Source: CAD feature listing. Evaluate the final solid. Frame: model axes, mm. A direction names the side the tool comes from. Coordinates: 2 decimals unless noted, no trailing zeros. Order: outer loops, then holes, each group sorted by start corner. A loop starts at its lowest first (then second) coordinate and runs counter-clockwise, first axis right, second up.
```python
from build123d import *
from build123d import SkipClean  # not in build123d's __all__

# Parameters (mm, degrees)
F1_DEPTH    = 28
F2_T1_DEPTH = 28
F2_T3_DEPTH = 31.2745707181
F3_R        = 14
F4_DEPTH    = 4
F6_DEPTH    = 2.5
F7_R        = 3.25
F8_DEPTH    = 31.3042238242
F9_R        = 7.5
F10_DEPTH   = 24.8042238242
F11_R       = 6.5
F12_DEPTH   = 4
F13_W       = 4
F13_H       = 21.4542382136
F14_DEPTH   = 2.5
F15_W       = 14
F15_H       = 21.4542382136
F16_DEPTH   = 1.2
F18_DEPTH   = 14


# Not quite as in the source:
# - a fillet or chamfer that OpenCascade refuses, or shapes differently, is made with other operations: its cross-section is extruded or revolved along the edge and cut away or added


with BuildPart() as f1:
    # F0 (on Right) → F1 (new body)
    with BuildSketch(Plane.YZ):
        with BuildLine():
            Line((0, 0), (-32, 0))
            Line((-32, 0), (-32, -2.5))
            Line((-32, -2.5), (0, -2.5))
            ThreePointArc((0, -2.5), (7.0205462081, 3.6568537819), (1.8327303277, 11.4209689242))
            Line((1.8327303277, 11.4209689242), (-31.8381916428, 20.4430652746))
            Line((-31.8381916428, 20.4430652746), (-56.5658795558, 24.8032238242))
            Line((-56.5658795558, 24.8032238242), (-57, 22.3412044417))
            Line((-57, 22.3412044417), (-32.3798061747, 18))
            Line((-32.3798061747, 18), (1.1856827149, 9.0061543585))
            ThreePointArc((1.1856827149, 9.0061543585), (4.5419340547, 3.9831692624), (0, 0))
        make_face()
    extrude(amount=F1_DEPTH)

    # F2: fillet of radius 15 on 2 edges, made by hand

    # F2_s2 → F2_t1 (join)
    with BuildSketch(Plane.YZ):
        with BuildLine():
            ThreePointArc((-33.0247707009, 18.1137246476), (-32.3828991568, 17.9860484592), (-31.7472076894, 17.8304957467))
            Line((-31.7472076894, 17.8304957467), (-32.3798061747, 18))
            Line((-32.3798061747, 18), (-33.0247707009, 18.1137246476))
        make_face()
    extrude(amount=F2_T1_DEPTH)

    # F2_s4 → F2_t3 (cut)
    with BuildSketch(Plane.YZ.offset(-1.6372853591)):
        with BuildLine():
            ThreePointArc((-31.2055931575, 20.2735610213), (-31.841284625, 20.4291137338), (-32.483156169, 20.5567899222))
            Line((-32.483156169, 20.5567899222), (-31.8381916428, 20.4430652746))
            Line((-31.8381916428, 20.4430652746), (-31.2055931575, 20.2735610213))
        make_face()
    extrude(amount=F2_T3_DEPTH, mode=Mode.SUBTRACT)

    # F3 (on face) → F4 (join)
    with BuildSketch(Plane(origin=(0, 0, -2.5), x_dir=(1, 0, 0), z_dir=(0, 0, -1))):
        with Locations((14, 18)):
            Circle(F3_R)
    extrude(amount=F4_DEPTH)

    # F5 (on face) → F6 (cut, through all)
    with BuildSketch(Plane(origin=(0, 0, -2.5), x_dir=(1, 0, 0), z_dir=(0, 0, -1))):
        with BuildLine():
            ThreePointArc((0, 18), (4.1005050634, 27.8994949366), (14, 32))
            Line((14, 32), (0, 32))
            Line((0, 32), (0, 18))
        make_face()
        with BuildLine():
            Line((28, 18), (28, 32))
            Line((28, 32), (14, 32))
            ThreePointArc((14, 32), (23.8994949366, 27.8994949366), (28, 18))
        make_face()
    with SkipClean():  # cleaning this boolean's faces spoils the solid; the shape is the same uncleaned
        extrude(amount=-F6_DEPTH, mode=Mode.SUBTRACT)

    # F7 (on face) → F8 (cut, through all)
    with BuildSketch(Plane(origin=(0, 0, -6.5), x_dir=(1, 0, 0), z_dir=(0, 0, -1))):
        with Locations((14, 18)):
            Circle(F7_R)
    with SkipClean():  # cleaning this boolean's faces spoils the solid; the shape is the same uncleaned
        extrude(amount=-F8_DEPTH, mode=Mode.SUBTRACT)

    # F9 (on face) → F10 (cut, through all)
    with BuildSketch(Plane.XY):
        with Locations((14, -18)):
            Circle(F9_R)
    with SkipClean():  # cleaning this boolean's faces spoils the solid; the shape is the same uncleaned
        extrude(amount=F10_DEPTH, mode=Mode.SUBTRACT)

    # F11 (on face) → F12 (cut)
    with BuildSketch(Plane.XY):
        with Locations((14, -18)):
            Circle(F11_R)
    with SkipClean():  # cleaning this boolean's faces spoils the solid; the shape is the same uncleaned
        extrude(amount=-F12_DEPTH, mode=Mode.SUBTRACT)

    # F13 (on face) → F14 (cut, through all)
    with BuildSketch(Plane(origin=(0, 2.5359311092, 14.3819799952), x_dir=(1, 0, 0), z_dir=(0, 0.1736481777, 0.984807753))):
        with Locations((23, -49.2864322531)):
            Rectangle(F13_W, F13_H)
        with Locations((5, -49.2864322531)):
            Rectangle(F13_W, F13_H)
    with SkipClean():  # cleaning this boolean's faces spoils the solid; the shape is the same uncleaned
        extrude(amount=-F14_DEPTH, mode=Mode.SUBTRACT)

    # F15 (on face) → F16 (cut)
    with BuildSketch(Plane(origin=(0, 2.5359311092, 14.3819799952), x_dir=(1, 0, 0), z_dir=(0, 0.1736481777, 0.984807753))):
        with Locations((14, -49.2864322531)):
            Rectangle(F15_W, F15_H)
    with SkipClean():  # cleaning this boolean's faces spoils the solid; the shape is the same uncleaned
        extrude(amount=-F16_DEPTH, mode=Mode.SUBTRACT)

    # F17 (on face) → F18 (join, through all)
    with BuildSketch(Plane(origin=(7, 0, 0), x_dir=(0, -1, 0), z_dir=(-1, 0, 0))):
        Polygon((53.5699966888, 25.0873101332), (53.9172930442, 23.1176946272), (56.774257369, 23.6214545206), (54.7517659925, 25.2956879464), align=None)
    with SkipClean():  # cleaning this boolean's faces spoils the solid; the shape is the same uncleaned
        extrude(amount=-F18_DEPTH)


solid = f1.part
```
Q1. Pull-direction query (Y, two-part tool) for faces 1 (the flat face through (13.804, -45.18, 20.257)), 2 (the flat face through (10.69, -10.78, 14.8)), 3 (the flat face through (13.846, -35.603, 20.138)); classes: pulls with the +Y half, pulls with the -Y half, needs draft (parallel to the pull), parting line crosses it, or undercut.
Solutions:
face 1: pulls with the -Y half
face 2: pulls with the +Y half
face 3: undercut
Q2. Set-up query: faces 4 (the flat face through (20.03, -11.85, 12.5)), 5 (the flat face through (12, -15, -4)), 6 (the flat face through (13.902, -55.777, 24.447)), 7 (the flat face through (14, -3, -2.5)). Return all of +Z, -Z, +X, -X, +Y, -Y with unobstructed straight access to the full face (end or side cutting, diameter ignored); none if empty.
Solutions:
face 4: +X, -X, -Y
face 5: +Z
face 6: +Z, -Y
face 7: -Z, +Y
Q3. Material intervals for line 1 along Y through (x, z) = (14, -4.7); line 2 along Z through (x, y) = (10.5, -24); line 3 along Z through (x, y) = (5.25, -28), sorted ascending.
Solutions:
line 1: y = -32 to -21.25, -14.75 to -4
line 2: z = -6.5 to 0
line 3: z = -6.5 to 0, 16.83 to 19.41
Q4. Section query B-B on x = 19.5. Output: boundary loops of the cut face in (y, z).
Solutions:
outline: (-57, 22.34) - (-33.02, 18.11) arc R15 cw to (-31.75, 17.83) - (-23.1, 15.51) - (-23.1, 18.1) - (-31.21, 20.27) arc R15 ccw to (-32.48, 20.56) - (-35.44, 21.08) - (-35.65, 19.9) - (-53.92, 23.12) - (-53.57, 25.09) - (-54.75, 25.3) - (-56.77, 23.62) - close; (-30.87, -6.5) - (-5.13, -6.5) - (-5.13, -2.5) - (0, -2.5) arc R7.08 ccw to (1.83, 11.42) - (-12.9, 15.37) - (-12.9, 12.78) - (1.19, 9.01) arc R4.58 cw to (0, 0) - (-14.54, 0) - (-14.54, -4) - (-21.46, -4) - (-21.46, 0) - (-30.87, 0) - close
Q5. Pin query (flat end, axial travel): P1, Ø14.5, axis at x = 13, y = -15.5, coming from the +Z side; P2, Ø6, axis at x = 20.5, y = -42, coming from the +Z side; P3, Ø8.5, axis at x = 15.5, y = -21, coming from the +Z side. Return the tip coordinate at first contact, or that it passes through.
Solutions:
P1: stops at z = 16.95
P2: stops at z = 21.55
P3: stops at z = 18.67
Q6. Section query D-D on x = 23. Output: boundary loops of the cut face in (y, z), plus the area to 3 significant figures.
Solutions:
outline: (-35.87, 18.62) - (-33.02, 18.11) arc R15 cw to (-31.75, 17.83) - (1.19, 9.01) arc R4.58 cw to (0, 0) - (-28.72, 0) - (-28.72, -6.5) - (-7.28, -6.5) - (-7.28, -2.5) - (0, -2.5) arc R7.08 ccw to (1.83, 11.42) - (-31.21, 20.27) arc R15 ccw to (-32.48, 20.56) - (-35.44, 21.08) - close
area: 296 mm2
Q7. Section query A-A on y = -39. Output: boundary loops of the cut face in (x, z).
Solutions:
outline: (0, 19.17) - (3, 19.17) - (3, 21.71) - (0, 21.71) - close; (7, 19.17) - (21, 19.17) - (21, 20.49) - (7, 20.49) - close; (25, 19.17) - (28, 19.17) - (28, 21.71) - (25, 21.71) - close
Q8. Section query C-C on y = -16.5. Output: boundary loops of the cut face in (x, z).
Solutions:
outline: (0, -2.5) - (0.08, -2.5) - (0.08, -6.5) - (11.12, -6.5) - (11.12, -4) - (7.68, -4) - (7.68, 0) - (0, 0) - close; (0, 13.75) - (6.65, 13.75) - (6.65, 16.33) - (0, 16.33) - close; (16.88, -6.5) - (27.92, -6.5) - (27.92, -2.5) - (28, -2.5) - (28, 0) - (20.32, 0) - (20.32, -4) - (16.88, -4) - close; (21.35, 13.75) - (28, 13.75) - (28, 16.33) - (21.35, 16.33) - close
